Could you check a few things on this model? Use its own coordinates, in mm. Face numbers are marked on the shaded views. A direction names the side the tool comes from. Coordinates: 2 decimals unless noted, no trailing zeros. Order: outer loops, then holes, each group sorted by start corner. A loop starts at its lowest first (then second) coordinate and runs counter-clockwise, first axis right, second up. Notation, with made-up numbers: (18, 33.25) -> (44, 33.25) arc R7 ccw to (44, 40.25) -> close; hole circle Ø8 at (2, 11.25). An arc over 180 degrees is marked (long way). Return JSON: item names as keys, results as strings. Group by question number.
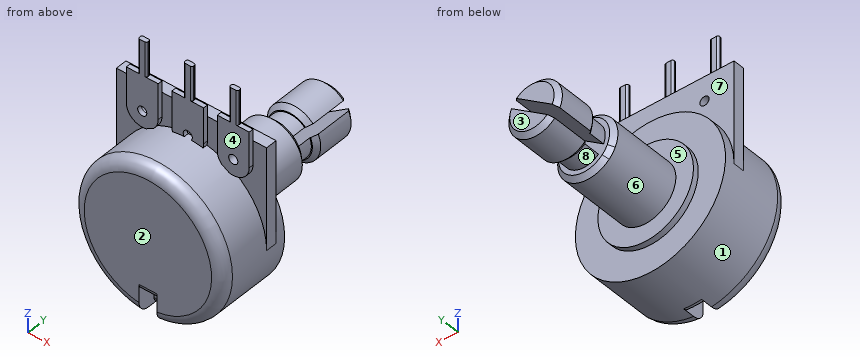
from build123d import *

# Parameters (mm, degrees)
SKETCH2_W           = 16.764
SKETCH2_H           = 1.27
BOSS_EXTRUDE1_DEPTH = 11.43
SKETCH3_R           = 0.508
BOSS_EXTRUDE2_DEPTH = 0.508
SKETCH5_R           = 8.382
SKETCH5_R_2         = 5.334
CUT_EXTRUDE2_DEPTH  = 15.875
LPATTERN1_COUNT     = 2
LPATTERN1_PITCH     = 5.08
LPATTERN2_COUNT     = 2
LPATTERN2_PITCH     = 5.08
SKETCH7_R           = 0.508
CUT_EXTRUDE3_DEPTH  = 1.27
CUT_EXTRUDE4_DEPTH  = 6.985
CHAMFER1_SIZE       = 0.508
FILLET1_R           = 1.27
FILLET2_R           = 0.2
SKETCH9_W           = 2
SKETCH9_H           = 3.195606775
CUT_EXTRUDE5_DEPTH  = 2
FILLET3_R           = 0.6


with BuildPart() as part:
    # Sketch1 → Base-Revolve (revolve)
    with BuildSketch(Plane.XY):
        Polygon((0, 0), (8.382, 0), (8.382, 8.89), (3.3655, 8.89), (3.3655, 17.145), (2.3622, 17.145), (2.3622, 19.05), (2.9845, 19.05), (2.9845, 24.13), (0, 24.13), align=None)
    revolve(axis=Axis((0, 0, 0), (0, -1, 0)))

    # Sketch2 → Boss-Extrude1 (add)
    with BuildSketch(Plane.XY):
        with Locations((0, 6.477)):
            Rectangle(SKETCH2_W, SKETCH2_H)
    extrude(amount=BOSS_EXTRUDE1_DEPTH)

    # Sketch3 → Boss-Extrude2 (add)
    with BuildSketch(Plane.XZ.offset(-5.842)):
        with BuildLine():
            Line((-1.778, 12.7), (-0.4826, 12.7))
            Line((-0.4826, 12.7), (-0.4826, 16.5608))
            Line((-0.4826, 16.5608), (0.4826, 16.5608))
            Line((0.4826, 16.5608), (0.4826, 12.7))
            Line((0.4826, 12.7), (1.778, 12.7))
            Line((1.778, 12.7), (1.778, 8.7122))
            ThreePointArc((1.778, 8.7122), (0, 6.9342), (-1.778, 8.7122))
            Line((-1.778, 8.7122), (-1.778, 12.7))
        make_face()
        with Locations((0, 8.7122)):
            Circle(SKETCH3_R, mode=Mode.SUBTRACT)
    boss_extrude2 = extrude(amount=BOSS_EXTRUDE2_DEPTH)

    # Sketch5 → Cut-Extrude2 (cut)
    with BuildSketch(Plane(origin=(0, 24.13, 0), x_dir=(-1, 0, 0), z_dir=(0, 1, 0))):
        Circle(SKETCH5_R)
        Circle(SKETCH5_R_2, mode=Mode.SUBTRACT)
    extrude(amount=-CUT_EXTRUDE2_DEPTH, mode=Mode.SUBTRACT)

    # LPattern1: Boss-Extrude2 ×2
    with Locations(*[(-i * LPATTERN1_PITCH, 0, 0) for i in range(1, LPATTERN1_COUNT)]):
        add(boss_extrude2)

    # LPattern2: Boss-Extrude2 ×2
    with Locations(*[(i * LPATTERN2_PITCH, 0, 0) for i in range(1, LPATTERN2_COUNT)]):
        add(boss_extrude2)

    # Sketch7 → Cut-Extrude3 (cut)
    with BuildSketch(Plane.XZ.offset(-5.842)):
        with Locations((-5.08, 8.7122)):
            Circle(SKETCH7_R)
        with Locations((0, 8.7122)):
            Circle(SKETCH7_R)
        with Locations((5.08, 8.7122)):
            Circle(SKETCH7_R)
    extrude(amount=-CUT_EXTRUDE3_DEPTH, mode=Mode.SUBTRACT)

    # Sketch8 → Cut-Extrude4 (cut)
    with BuildSketch(Plane(origin=(0, 24.13, 0), x_dir=(-1, 0, 0), z_dir=(0, 1, 0))):
        with BuildLine():
            Line((-2.708292046, 1.253951532), (2.13071284, -2.089809331))
            ThreePointArc((2.13071284, -2.089809331), (2.455332287, -1.696638916), (2.708292046, -1.253951532))
            Line((2.708292046, -1.253951532), (-2.13071284, 2.089809331))
            ThreePointArc((-2.13071284, 2.089809331), (-2.455332287, 1.696638916), (-2.708292046, 1.253951532))
        make_face()
    extrude(amount=-CUT_EXTRUDE4_DEPTH, mode=Mode.SUBTRACT)

    # Chamfer1
    chamfer1_edges = [part.edges().sort_by_distance(p)[0] for p in [
        (1.128744386, 24.13, -2.762820364),
        (-1.696638916, 24.13, 2.455332287),
        (1.128744386, 19.05, -2.762820364),
        (-1.696638916, 19.05, 2.455332287),
        (-3.3655, 17.145, 0),
    ]]
    chamfer(chamfer1_edges, length=CHAMFER1_SIZE)

    # Fillet1
    fillet1_edges = [part.edges().sort_by_distance(p)[0] for p in [
        (-8.382, 0, 0),
    ]]
    fillet(fillet1_edges, radius=FILLET1_R)

    # Fillet2
    fillet2_edges = [part.edges().sort_by_distance(p)[0] for p in [
        (4.5974, 5.842, 14.6304),
        (5.5626, 5.842, 14.6304),
        (5.5626, 5.334, 14.6304),
        (4.5974, 5.334, 14.6304),
        (-0.4826, 5.842, 14.6304),
        (0.4826, 5.842, 14.6304),
        (0.4826, 5.334, 14.6304),
        (-0.4826, 5.334, 14.6304),
        (-5.5626, 5.842, 14.6304),
        (-4.5974, 5.842, 14.6304),
        (-4.5974, 5.334, 14.6304),
        (-5.5626, 5.334, 14.6304),
    ]]
    fillet(fillet2_edges, radius=FILLET2_R)

    # Sketch9 → Cut-Extrude5 (cut)
    with BuildSketch(Plane.XZ):
        with Locations((0, -7.204164856)):
            Rectangle(SKETCH9_W, SKETCH9_H)
    extrude(amount=-CUT_EXTRUDE5_DEPTH, mode=Mode.SUBTRACT)

    # Fillet3
    fillet3_edges = [part.edges().sort_by_distance(p)[0] for p in [
        (0, 2, -8.382),
        (0, 0, -5.606361468),
        (0, 2, -5.606361468),
    ]]
    fillet(fillet3_edges, radius=FILLET3_R)


solid = part.part
Q1. I want a section at A-A on z = 13.25. Please give me the cut outline in (x, y), and give its area (3 significant figures).
Q2. On a 3-axis mill with a long thin cutter (end or side, diameter ignored), from which of +Z, -Z, +X, -X, +Y, -Y can I reach the whole of each face in a straight line? I mean the marked faces 1, 2, 3, 4 and 5. Say none if no direction works.
Q3. I'm going to push flat-ended pins straight in: pin 1 Ø1.8 at (x, z) = (-4, 13.5) entering from -Y; pin 2 Ø0.6 at (y, z) = (5.5, 11) entering from -X; pin 3 Ø4 at (x, z) = (-4, 15) entering from +Y. Where does each tip first touch, or does it pass through?
Q4. I want a section at B-B on y = 22.75. Please give me the cut outline in (x, z).
Q5. I need wall thicknesses on line 1 along Z through (x, y) = (0, 5.75); line 2 along Z through (x, y) = (-5.08, 5.65); line 3 along Y through (x, z) = (-3.25, -5.25) (3 decimals). Which ranges of each line are inside material? Lowest first, please. Write a range as from..to.
Q6. I want a section at D-D on y = 10.25. Please give me the cut outline in (x, z), and give its area (3 significant figures).
Q7. We'd pull the mould along Y, two halves only. Please class the marked faces 6, 7 and 8: pulls with the +Y half, pulls with the -Y half, needs draft (parallel to the pull), parting line crosses it, or undercut.
Q8. I want a section at C-C on y = 3.25. Please give me the cut outline in (x, z).
Response values:
{
 "1": {"outline": "(-5.56, 5.53) arc R0.2 ccw to (-5.36, 5.33) -> (-4.8, 5.33) arc R0.2 ccw to (-4.6, 5.53) -> (-4.6, 5.64) arc R0.2 ccw to (-4.8, 5.84) -> (-5.36, 5.84) arc R0.2 ccw to (-5.56, 5.64) -> close; (-0.48, 5.53) arc R0.2 ccw to (-0.28, 5.33) -> (0.28, 5.33) arc R0.2 ccw to (0.48, 5.53) -> (0.48, 5.64) arc R0.2 ccw to (0.28, 5.84) -> (-0.28, 5.84) arc R0.2 ccw to (-0.48, 5.64) -> close; (4.6, 5.53) arc R0.2 ccw to (4.8, 5.33) -> (5.36, 5.33) arc R0.2 ccw to (5.56, 5.53) -> (5.56, 5.64) arc R0.2 ccw to (5.36, 5.84) -> (4.8, 5.84) arc R0.2 ccw to (4.6, 5.64) -> close", "area": "1.37 mm²"},
 "2": {"face 1": "none", "face 2": "+Z, -Z, +X, -X, -Y", "face 3": "+Z, -Z, +X, -X, +Y", "face 4": "+Z, +X, -Y", "face 5": "+Y"},
 "3": {"pin 1": "stops at y = 5.33", "pin 2": "stops at x = -6.86", "pin 3": "stops at y = 5.84"},
 "4": {"outline": "(-2.71, -1.25) -> (2.13, 2.09) arc R2.98 ccw to start; (-2.13, -2.09) arc R2.98 ccw to (2.71, 1.25) -> close"},
 "5": {"line 1": "z = -8.38..8.38, 9.22..16.56", "line 2": "z = -6.67..6.67, 6.93..8.2, 9.22..16.56", "line 3": "y = 0..8.255"},
 "6": {"outline": "circle Ø6.73 at (0, 0)", "area": "35.6 mm²"},
 "7": {"face 6": "needs draft", "face 7": "pulls with the +Y half", "face 8": "undercut"},
 "8": {"outline": "circle Ø16.76 at (0, 0)"}
}
